Autodesk Inventor part; units mm, degrees
ref_plane "YZ Plane" through (0, 0, 0) normal (1, 0, 0) x (0, 1, 0)
ref_plane "XZ Plane" through (0, 0, 0) normal (0, 1, 0) x (-1, 0, 0)
ref_plane "XY Plane" through (0, 0, 0) normal (0, 0, 1) x (1, 0, 0)
sketch "Sketch1" plane through (0, 0, 0) normal (0, 0, 1) x (1, 0, 0)
  line L0 (0, 0) -> (7, 0)
  line L1 (7, 0) -> (7, 20)
  line L2 (7, 20) -> (0, 20)
  line L3 (0, 20) -> (0, 0)
  line L4 (7, 20) -> (27, 20)
  line L5 (27, 20) -> (27, 13)
  line L6 (27, 13) -> (7, 13)
  line L7 (7, 13) -> (7, 20)
  line L8 (27, 20) -> (34, 20)
  line L9 (34, 20) -> (34, 0)
  line L10 (34, 0) -> (27, 0)
  line L11 (27, 0) -> (27, 20)
  dimension "d0" = 34
  dimension "d1" = 7
  dimension "d2" = 7
  dimension "d3" = 7
  dimension "d4" = 13
extrude "Extrusion1" add sketch "Sketch1" along normal blind 20
sketch "Sketch2" plane through (7, 0, 0) normal (1, 0, 0) x (0, 0, -1)
  circle A0 centre (-10, 5) radius 2.5
  line L0 (-20, 0) -> (-20, 20)
  line L1 (0, 0) -> (-20, 0)
  dimension "d7" = 5
  dimension "d8" = 10
  dimension "d9" = 5
extrude "Extrusion2" cut sketch "Sketch2" along normal blind 60 and the other way blind 10
properties part number "FanSpace"
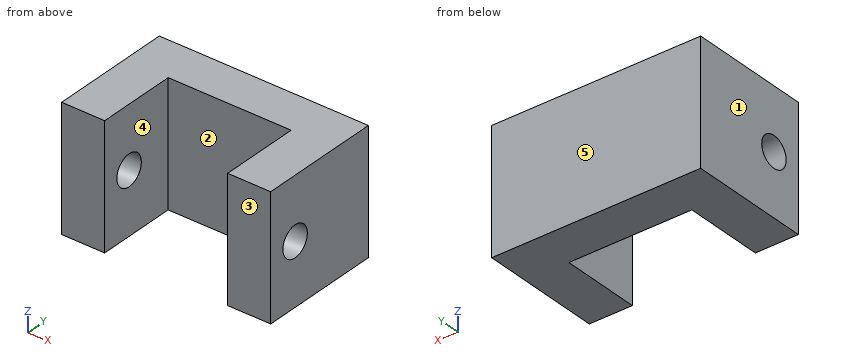
Part model, mm, in its own coordinate system. Face numbers are marked on the shaded views. A direction names the side the tool comes from. Coordinates: 2 decimals unless noted, no trailing zeros. Order: outer loops, then holes, each group sorted by start corner. A loop starts at its lowest first (then second) coordinate and runs counter-clockwise, first axis right, second up. Notation, with made-up numbers: (-40, 10) -> (-17, 10) arc R36 cw to (-17, 49) -> close; hole circle Ø1 at (61, 30). An arc over 180 degrees is marked (long way). Put each result on its own line as item: value. Start each with the question number.
(1) Band-saw the part on D-D (y = 5). Give the cut face in (x, z), then the cut area to 3 significant figures.
(2) Band-saw the part on C-C (x = 6). Give the cut face in (y, z), then the cut area to 3 significant figures.
(3) Pin check, flat tips, straight feed: pin 1 Ø8 at (y, z) = (16.5, 4) entering from -X; pin 2 Ø1 at (x, z) = (12, 10.5) entering from -Y. Stop position of each tip, or through.
(4) Band-saw the part on B-B (y = 8). Give the cut face in (x, z).
(5) Probe line 1 along X through (y, z) = (2.25, 2.75); line 2 along Z through (x, y) = (29.5, 5); line 3 along Y through (x, z) = (31, 10). List the from-to ranges inside material, lowest first. Write a range as [from, to].
(6) Mould opens along X. For the marked faces 1, 2 and 3 say: pulls with the +X half, pulls with the -X half, needs draft (parallel to the pull), parting line crosses it, or undercut.
(7) Which spindle directions (+Z, -Z, +X, -X, +Y, -Y) get a long thin tool onto all of the face, cutting with end or side? Do the marked faces 4 and 5. Say none if no direction does.
(8) Band-saw the part on A-A (z = 10). Give the cut face in (x, y).
Determined:
1. outline: (0, 0) -> (7, 0) -> (7, 7.5) -> (0, 7.5) -> close; (0, 12.5) -> (7, 12.5) -> (7, 20) -> (0, 20) -> close; (27, 0) -> (34, 0) -> (34, 7.5) -> (27, 7.5) -> close; (27, 12.5) -> (34, 12.5) -> (34, 20) -> (27, 20) -> close
1. area: 210 mm²
2. outline: (0, 0) -> (20, 0) -> (20, 20) -> (0, 20) -> close; hole circle Ø5 at (5, 10)
2. area: 380 mm²
3. pin 1: stops at x = 0
3. pin 2: stops at y = 13
4. outline: (0, 0) -> (7, 0) -> (7, 20) -> (0, 20) -> close; (27, 0) -> (34, 0) -> (34, 20) -> (27, 20) -> close
5. line 1: x = [0, 7], [27, 34]
5. line 2: z = [0, 7.5], [12.5, 20]
5. line 3: y = [0, 2.5], [7.5, 20]
6. face 1: pulls with the -X half
6. face 2: undercut
6. face 3: needs draft
7. face 4: +Z, -Z, -Y
7. face 5: +Z, -Z, +X, -X, +Y
8. outline: (0, 0) -> (7, 0) -> (7, 2.5) -> (0, 2.5) -> close; (0, 7.5) -> (7, 7.5) -> (7, 13) -> (27, 13) -> (27, 7.5) -> (34, 7.5) -> (34, 20) -> (0, 20) -> close; (27, 0) -> (34, 0) -> (34, 2.5) -> (27, 2.5) -> close
